```python
from build123d import *

# Parameters (mm, degrees)
SKETCH1_R           = 1.5
BOSS_EXTRUDE1_DEPTH = 10
SKETCH2_W           = 20.5
SKETCH2_H           = 145
CUT_EXTRUDE1_DEPTH  = 5
SKETCH3_W           = 20
SKETCH3_H           = 25
CUT_EXTRUDE2_DEPTH  = 181.969610709
SKETCH4_W           = 50
SKETCH4_H           = 3
CUT_EXTRUDE3_DEPTH  = 5
FILLET1_R           = 3
SKETCH6_R           = 1.5
CUT_EXTRUDE4_DEPTH  = 5
CHAMFER2_SIZE       = 1


with BuildPart() as part:
    # Sketch1 → Boss-Extrude1 (new body)
    with BuildSketch(Plane(origin=(0, 0, 0), x_dir=(1, 0, 0), z_dir=(0, 1, 0))):
        with BuildLine():
            Line((0, -30), (0, 0))
            Line((0, 0), (-45, 0))
            Line((-45, 0), (-45, -10))
            Line((-45, -10), (-30, -92.5))
            Line((-30, -92.5), (-30, -175))
            Line((-30, -175), (0, -175))
            Line((0, -175), (0, -165))
            ThreePointArc((0, -165), (-2.828427125, -163.828427125), (-4, -161))
            Line((-4, -161), (-4, -34))
            ThreePointArc((-4, -34), (-2.828427125, -31.171572875), (0, -30))
        make_face()
        with Locations(Location((-40, -5, 0), (0, 0, 270))):
            Circle(SKETCH1_R, mode=Mode.SUBTRACT)
    boss_extrude1 = extrude(amount=BOSS_EXTRUDE1_DEPTH)

    # Sketch2 → Cut-Extrude1 (cut)
    with BuildSketch(Plane(origin=(0, 10, 0), x_dir=(1, 0, 0), z_dir=(0, 1, 0))):
        with Locations((-10.25, -97.5)):
            Rectangle(SKETCH2_W, SKETCH2_H)
    cut_extrude1 = extrude(amount=-CUT_EXTRUDE1_DEPTH, mode=Mode.SUBTRACT)

    # Mirror1: Boss-Extrude1, Cut-Extrude1 across plane
    add(boss_extrude1.mirror(Plane(origin=(0, 0, 0), x_dir=(0, 0, 1), z_dir=(1, 0, 0))))
    add(cut_extrude1.mirror(Plane(origin=(0, 0, 0), x_dir=(0, 0, 1), z_dir=(1, 0, 0))), mode=Mode.SUBTRACT)

    # Sketch3 → Cut-Extrude2 (cut, through all)
    with BuildSketch(Plane(origin=(0, 10, 0), x_dir=(1, 0, 0), z_dir=(0, 1, 0))):
        with Locations((0, -12.5)):
            Rectangle(SKETCH3_W, SKETCH3_H)
    extrude(amount=-CUT_EXTRUDE2_DEPTH, mode=Mode.SUBTRACT)

    # Sketch4 → Cut-Extrude3 (cut)
    with BuildSketch(Plane(origin=(0, 10, 0), x_dir=(1, 0, 0), z_dir=(0, 1, 0))):
        with Locations((0, -10)):
            Rectangle(SKETCH4_W, SKETCH4_H)
    extrude(amount=-CUT_EXTRUDE3_DEPTH, mode=Mode.SUBTRACT)

    # Fillet1
    # the kernel refuses this fillet: 3 mm, written as the material it takes off along each edge
    with BuildSketch(Plane(origin=(-63, 10, 0), x_dir=(0, -1, 0), z_dir=(1, 0, 0)), Plane(origin=(-8, 10, 0), x_dir=(0, -1, 0), z_dir=(1, 0, 0))) as fillet1_piece_1:
        with BuildLine():
            CenterArc((FILLET1_R, -FILLET1_R), FILLET1_R, 90, 90)
            Line((0, -FILLET1_R), (-FILLET1_R * 0.02, -FILLET1_R))
            Line((-FILLET1_R * 0.02, -FILLET1_R), (-FILLET1_R * 0.02, FILLET1_R * 0.02))
            Line((-FILLET1_R * 0.02, FILLET1_R * 0.02), (FILLET1_R, FILLET1_R * 0.02))
            Line((FILLET1_R, FILLET1_R * 0.02), (FILLET1_R, 0))
        make_face()
    extrude(amount=71, mode=Mode.SUBTRACT)
    with BuildSketch(Plane(origin=(-48.219937888, 10, -7.709658382), x_dir=(0, -1, 0), z_dir=(0.1788854381999831, 0, 0.9838699100999075))) as fillet1_piece_2_section:
        with BuildLine():
            CenterArc((FILLET1_R, FILLET1_R), FILLET1_R, 180, 90)
            Line((0, FILLET1_R), (-FILLET1_R * 0.02, FILLET1_R))
            Line((-FILLET1_R * 0.02, FILLET1_R), (-FILLET1_R * 0.02, -FILLET1_R * 0.02))
            Line((-FILLET1_R * 0.02, -FILLET1_R * 0.02), (FILLET1_R, -FILLET1_R * 0.02))
            Line((FILLET1_R, -FILLET1_R * 0.02), (FILLET1_R, 0))
        make_face()
    fillet1_piece_2 = extrude(amount=119.852549156, mode=Mode.PRIVATE)
    fillet1_piece_2 = split(fillet1_piece_2, bisect_by=Plane(origin=(-30, 9.306962758, 40.50367668), z_dir=(-1, 0, 0)), keep=Keep.TOP, mode=Mode.PRIVATE)
    add(fillet1_piece_2, mode=Mode.SUBTRACT)
    with BuildSketch(Plane(origin=(-30, 10, 74.5), x_dir=(0, -1, 0), z_dir=(0, 0, 1))) as fillet1_piece_3_section:
        with BuildLine():
            CenterArc((FILLET1_R, FILLET1_R), FILLET1_R, 180, 90)
            Line((0, FILLET1_R), (-FILLET1_R * 0.02, FILLET1_R))
            Line((-FILLET1_R * 0.02, FILLET1_R), (-FILLET1_R * 0.02, -FILLET1_R * 0.02))
            Line((-FILLET1_R * 0.02, -FILLET1_R * 0.02), (FILLET1_R, -FILLET1_R * 0.02))
            Line((FILLET1_R, -FILLET1_R * 0.02), (FILLET1_R, 0))
        make_face()
    fillet1_piece_3 = extrude(amount=118.5, mode=Mode.PRIVATE)
    fillet1_piece_3 = split(fillet1_piece_3, bisect_by=Plane(origin=(-20.817808359, 9.30676914, 143.002054026), z_dir=(-0.9838699100999075, 0, 0.1788854381999831)), keep=Keep.TOP, mode=Mode.PRIVATE)
    add(fillet1_piece_3, mode=Mode.SUBTRACT)
    with BuildSketch(Plane(origin=(48, 10, 175), x_dir=(0, -1, 0), z_dir=(-1, 0, 0))) as fillet1_piece_4:
        with BuildLine():
            CenterArc((FILLET1_R, -FILLET1_R), FILLET1_R, 90, 90)
            Line((0, -FILLET1_R), (-FILLET1_R * 0.02, -FILLET1_R))
            Line((-FILLET1_R * 0.02, -FILLET1_R), (-FILLET1_R * 0.02, FILLET1_R * 0.02))
            Line((-FILLET1_R * 0.02, FILLET1_R * 0.02), (FILLET1_R, FILLET1_R * 0.02))
            Line((FILLET1_R, FILLET1_R * 0.02), (FILLET1_R, 0))
        make_face()
    extrude(amount=96, mode=Mode.SUBTRACT)
    with BuildSketch(Plane(origin=(30, 10, 74.5), x_dir=(0, -1, 0), z_dir=(0, 0, 1))) as fillet1_piece_5_section:
        with BuildLine():
            CenterArc((FILLET1_R, -FILLET1_R), FILLET1_R, 90, 90)
            Line((0, -FILLET1_R), (-FILLET1_R * 0.02, -FILLET1_R))
            Line((-FILLET1_R * 0.02, -FILLET1_R), (-FILLET1_R * 0.02, FILLET1_R * 0.02))
            Line((-FILLET1_R * 0.02, FILLET1_R * 0.02), (FILLET1_R, FILLET1_R * 0.02))
            Line((FILLET1_R, FILLET1_R * 0.02), (FILLET1_R, 0))
        make_face()
    fillet1_piece_5 = extrude(amount=118.5, mode=Mode.PRIVATE)
    fillet1_piece_5 = split(fillet1_piece_5, bisect_by=Plane(origin=(20.817808359, 9.30676914, 143.002054026), z_dir=(0.9838699100999075, 0, 0.1788854381999831)), keep=Keep.TOP, mode=Mode.PRIVATE)
    add(fillet1_piece_5, mode=Mode.SUBTRACT)
    with BuildSketch(Plane(origin=(48.219937888, 10, -7.709658382), x_dir=(0, -1, 0), z_dir=(-0.1788854381999831, 0, 0.9838699100999075))) as fillet1_piece_6_section:
        with BuildLine():
            CenterArc((FILLET1_R, -FILLET1_R), FILLET1_R, 90, 90)
            Line((0, -FILLET1_R), (-FILLET1_R * 0.02, -FILLET1_R))
            Line((-FILLET1_R * 0.02, -FILLET1_R), (-FILLET1_R * 0.02, FILLET1_R * 0.02))
            Line((-FILLET1_R * 0.02, FILLET1_R * 0.02), (FILLET1_R, FILLET1_R * 0.02))
            Line((FILLET1_R, FILLET1_R * 0.02), (FILLET1_R, 0))
        make_face()
    fillet1_piece_6 = extrude(amount=119.852549156, mode=Mode.PRIVATE)
    fillet1_piece_6 = split(fillet1_piece_6, bisect_by=Plane(origin=(30, 9.306962758, 40.50367668), z_dir=(1, 0, 0)), keep=Keep.TOP, mode=Mode.PRIVATE)
    add(fillet1_piece_6, mode=Mode.SUBTRACT)
    with BuildSketch(Plane(origin=(-30, 10, 74.5), x_dir=(0, -1, 0), z_dir=(0, 0, 1))) as fillet1_piece_7a_section:
        with BuildLine():
            CenterArc((FILLET1_R, FILLET1_R), FILLET1_R, 180, 90)
            Line((0, FILLET1_R), (-FILLET1_R * 0.02, FILLET1_R))
            Line((-FILLET1_R * 0.02, FILLET1_R), (-FILLET1_R * 0.02, -FILLET1_R * 0.02))
            Line((-FILLET1_R * 0.02, -FILLET1_R * 0.02), (FILLET1_R, -FILLET1_R * 0.02))
            Line((FILLET1_R, -FILLET1_R * 0.02), (FILLET1_R, 0))
        make_face()
    fillet1_piece_7a = extrude(amount=118.5, mode=Mode.PRIVATE)
    fillet1_piece_7a = split(fillet1_piece_7a, bisect_by=Plane(origin=(-31.178924404, 9.383343973, 86.015915779), z_dir=(0.9838699100999075, 0, -0.1788854381999831)), keep=Keep.TOP, mode=Mode.PRIVATE)
    with BuildSketch(Plane(origin=(-48.219937888, 10, -7.709658382), x_dir=(0, -1, 0), z_dir=(0.1788854381999831, 0, 0.9838699100999075))) as fillet1_piece_7b_section:
        with BuildLine():
            CenterArc((FILLET1_R, FILLET1_R), FILLET1_R, 180, 90)
            Line((0, FILLET1_R), (-FILLET1_R * 0.02, FILLET1_R))
            Line((-FILLET1_R * 0.02, FILLET1_R), (-FILLET1_R * 0.02, -FILLET1_R * 0.02))
            Line((-FILLET1_R * 0.02, -FILLET1_R * 0.02), (FILLET1_R, -FILLET1_R * 0.02))
            Line((FILLET1_R, -FILLET1_R * 0.02), (FILLET1_R, 0))
        make_face()
    fillet1_piece_7b = extrude(amount=119.852549156, mode=Mode.PRIVATE)
    fillet1_piece_7b = split(fillet1_piece_7b, bisect_by=Plane(origin=(-30, 9.383343973, 99.090387768), z_dir=(1, 0, 0)), keep=Keep.TOP, mode=Mode.PRIVATE)
    fillet1_piece_7 = fillet1_piece_7a & fillet1_piece_7b
    add(fillet1_piece_7, mode=Mode.SUBTRACT)
    with BuildSketch(Plane(origin=(48.219937888, 10, -7.709658382), x_dir=(0, -1, 0), z_dir=(-0.1788854381999831, 0, 0.9838699100999075))) as fillet1_piece_8a_section:
        with BuildLine():
            CenterArc((FILLET1_R, -FILLET1_R), FILLET1_R, 90, 90)
            Line((0, -FILLET1_R), (-FILLET1_R * 0.02, -FILLET1_R))
            Line((-FILLET1_R * 0.02, -FILLET1_R), (-FILLET1_R * 0.02, FILLET1_R * 0.02))
            Line((-FILLET1_R * 0.02, FILLET1_R * 0.02), (FILLET1_R, FILLET1_R * 0.02))
            Line((FILLET1_R, FILLET1_R * 0.02), (FILLET1_R, 0))
        make_face()
    fillet1_piece_8a = extrude(amount=119.852549156, mode=Mode.PRIVATE)
    fillet1_piece_8a = split(fillet1_piece_8a, bisect_by=Plane(origin=(30, 9.383343973, 99.090387768), z_dir=(-1, 0, 0)), keep=Keep.TOP, mode=Mode.PRIVATE)
    with BuildSketch(Plane(origin=(30, 10, 74.5), x_dir=(0, -1, 0), z_dir=(0, 0, 1))) as fillet1_piece_8b_section:
        with BuildLine():
            CenterArc((FILLET1_R, -FILLET1_R), FILLET1_R, 90, 90)
            Line((0, -FILLET1_R), (-FILLET1_R * 0.02, -FILLET1_R))
            Line((-FILLET1_R * 0.02, -FILLET1_R), (-FILLET1_R * 0.02, FILLET1_R * 0.02))
            Line((-FILLET1_R * 0.02, FILLET1_R * 0.02), (FILLET1_R, FILLET1_R * 0.02))
            Line((FILLET1_R, FILLET1_R * 0.02), (FILLET1_R, 0))
        make_face()
    fillet1_piece_8b = extrude(amount=118.5, mode=Mode.PRIVATE)
    fillet1_piece_8b = split(fillet1_piece_8b, bisect_by=Plane(origin=(31.178924404, 9.383343973, 86.015915779), z_dir=(-0.9838699100999075, 0, -0.1788854381999831)), keep=Keep.TOP, mode=Mode.PRIVATE)
    fillet1_piece_8 = fillet1_piece_8a & fillet1_piece_8b
    add(fillet1_piece_8, mode=Mode.SUBTRACT)

    # Sketch6 → Cut-Extrude4 (cut)
    # profile 1 of 2: a face of its own
    with BuildSketch(Plane.XZ):
        Polygon((-42.230176428, 2.993432508), (-39.377349792, 2.065326812), (-37.147173364, 4.071894304), (-37.769823572, 7.006567492), (-40.622650208, 7.934673188), (-42.852826636, 5.928105696), align=None)
        with Locations(Location((-40, 5, 0), (0, 0, 270))):
            Circle(SKETCH6_R, mode=Mode.SUBTRACT)
    # profile 2 of 2: a face of its own
    with BuildSketch(Plane.XZ):
        Polygon((37.056735483, 4.419315936), (39.031254892, 2.160716126), (41.974519409, 2.74140019), (42.943264517, 5.580684064), (40.968745108, 7.839283874), (38.025480591, 7.25859981), align=None)
        with Locations(Location((40, 5, 0), (0, 0, 270))):
            Circle(SKETCH6_R, mode=Mode.SUBTRACT)
    extrude(amount=-CUT_EXTRUDE4_DEPTH, mode=Mode.SUBTRACT)

    # Chamfer2
    chamfer2_edges = [part.edges().sort_by_distance(p)[0] for p in [
        (-40.80376311, 5, 2.52937966),
        (-42.541501532, 5, 4.460769102),
        (-41.737738422, 5, 6.931389442),
        (-39.19623689, 5, 7.47062034),
        (-37.458498468, 5, 5.539230898),
        (-38.262261578, 5, 3.068610558),
        (38.043995187, 5, 3.290016031),
        (37.541108037, 5, 5.838957873),
        (39.497112849, 5, 7.548941842),
        (41.956004813, 5, 6.709983969),
        (42.458891963, 5, 4.161042127),
        (40.502887151, 5, 2.451058158),
    ]]
    chamfer(chamfer2_edges, length=CHAMFER2_SIZE)


solid = part.part
```
The model under review builds one solid part; all positions refer to its coordinate system, in mm. A direction names the side the tool comes from. Coordinates: 2 decimals unless noted, no trailing zeros. Order: outer loops, then holes, each group sorted by start corner. A loop starts at its lowest first (then second) coordinate and runs counter-clockwise, first axis right, second up. Notation, with made-up numbers: M 86.5,15 L 118.5,15 A19 cw 118.5,19 Z; hole C 23,78.5 d8. An arc over 180 degrees is marked long. One line per question, with ' | ' between items.
(1) Machinability: for faces 4 (the face through (25, 8, 10)), 5 (the face through (-41.464, 7.465, 4.675)), which of the approach directions +Z, -Z, +X, -X, +Y, -Y give a long, thin tool a straight path to every point of the face, cutting with its end or side? Answer none if there is none.
Geometry results:
face 4: +Y | face 5: +Y, -Y
(2) Add section A-A, the plane y = 2. Write out the cut boundary in (x, z), then the cut area to 3 significant figures.
Geometry results:
outline: M -45,0 L -10,0 L -10,25 L 10,25 L 10,0 L 45,0 L 45,10 L 30,92.5 L 30,175 L -30,175 L -30,92.5 L -45,10 Z; hole M -42.85,5.93 L -42.23,2.99 L -39.38,2.07 L -37.15,4.07 L -37.77,7.01 L -40.62,7.93 Z; hole M -4,34 A4 ccw 4,34 L 4,161 A4 ccw -4,161 Z; hole M 37.06,4.42 L 39.03,2.16 L 41.97,2.74 L 42.94,5.58 L 40.97,7.84 L 38.03,7.26 Z | area: 10,400 mm²
(3) For probe 1 along X at (y, z) = (7.15, 5); probe 2 along X at (y, z) = (4, 92.5); probe 3 along X at (y, z) = (7, 9), list the stretches that pass through material, from the lowest coordinate up. Write a range as from..to.
Geometry results:
probe 1: x = -45..-41.5, -38.5..-10, 10..38.5, 41.5..45 | probe 2: x = -30..-4, 4..30 | probe 3: x = -45..-25, 25..45
(4) Add section B-B, the plane x = 17. Write out the cut boundary in (y, z).
Geometry results:
outline: M 0,0 L 7,0 A3 ccw 10,3 L 10,8.5 L 5,8.5 L 5,11.5 L 10,11.5 L 10,25 L 5,25 L 5,170 L 10,170 L 10,172 A3 ccw 7,175 L 0,175 Z
(5) The part is to be moulded in two halves that separate along X. For faces 1 (the face through (0, 3, 25)), 2 (the face through (-45, 5, 5)), 3 (the face through (30, 3, 133)), say which applies: +X half, -X half, draft (parallel to the pull), parting line (faces both ways), or undercut.
Geometry results:
face 1: undercut | face 2: -X half | face 3: +X half
(6) Insertion check: pin 1 (6 mm diameter, centred on y = 8.5, z = 74.5, fed in from +X); pin 2 (3.5 mm diameter, centred on y = 4, z = 126, fed in from +X); pin 3 (12 mm diameter, centred on x = 19, z = 132.5, fed in from +Y); pin 4 (1.5 mm diameter, centred on y = 2, z = 21.5, fed in from +X). Each pin has a flat end and moves straight along its axis. Give the tip position at first contact, or say it passes through.
Geometry results:
pin 1: stops at x = 33.76 | pin 2: stops at x = 30 | pin 3: stops at y = 10 | pin 4: stops at x = 43.05
